```python
from build123d import *

# Parameters (mm, degrees)
SKETCH1_R           = 125
BOSS_EXTRUDE1_DEPTH = 5
SKETCH1_5_R         = 17.5
CUT_EXTRUDE4_DEPTH  = 10


with BuildPart() as part:
    # Sketch1 → Boss-Extrude1 (new body)
    with BuildSketch(Plane(origin=(0, 0, 0), x_dir=(1, 0, 0), z_dir=(0, 1, 0))):
        Circle(SKETCH1_R)
    extrude(amount=BOSS_EXTRUDE1_DEPTH)

    # Sketch1<5> → Cut-Extrude4 (cut)
    with BuildSketch(Plane(origin=(0, 0, 0), x_dir=(1, 0, 0), z_dir=(0, 1, 0))):
        with Locations((25.339393539, 77.986634336)):
            Circle(SKETCH1_5_R)
        with Locations((66.339393539, 48.198390688)):
            Circle(SKETCH1_5_R)
        with Locations((82, 0)):
            Circle(SKETCH1_5_R)
        with Locations((66.339393539, -48.198390688)):
            Circle(SKETCH1_5_R)
        with Locations((25.339393539, -77.986634336)):
            Circle(SKETCH1_5_R)
    extrude(amount=CUT_EXTRUDE4_DEPTH, mode=Mode.SUBTRACT)


solid = part.part
```
Can you work these out from the model? Positions are in its coordinate system, mm. Give positions to 0.01 mm unless a question says otherwise; leave off trailing zeros. Write each loop counter-clockwise with the first axis right and the second up, starting at its lowest first coordinate (ties: lowest second). Pieces come first, ordered by that corner, then holes. Notation, with made-up numbers: (30, -21.75) -> (84, -21.75) arc R18 ccw to (84, -8.75) -> close; hole circle Ø9 at (66, -28). An arc over 180 degrees is marked (long way). One line per item, written item: value.
Q1. Imagine slicing it at B-B on y = 2.95. Please give me the cut outline in (x, z), and give its area (3 significant figures).
Results found:
outline: circle Ø250 at (0, 0); hole circle Ø35 at (25.34, -77.99); hole circle Ø35 at (25.34, 77.99); hole circle Ø35 at (66.34, -48.2); hole circle Ø35 at (66.34, 48.2); hole circle Ø35 at (82, 0)
area: 44,300 mm^2
Q2. For P1, Ø1.5, axis at x = -38, y = 2.5, coming from the -Z side; P2, Ø21, axis at x = 25.34, z = -77.99, coming from the +Y side (3 decimals); P3, Ø3, axis at x = 21, y = 1, coming from the +Z side, each with a flat end and sliding along its axis, tell me the tip position at first contact or that it passes through.
Results found:
P1: stops at z = -119.32
P2: passes through
P3: stops at z = 123.47
Q3. Imagine slicing it at D-D on x = -43. Please give me the cut outline in (y, z).
Results found:
outline: (0, -117.37) -> (5, -117.37) -> (5, 117.37) -> (0, 117.37) -> close
Q4. Please list where these lines run through material, in increasing order: line 1 (X direction, y = 0.6, z = -63); line 2 (Z direction, x = 82, y = 1.2); line 3 (Z direction, x = 55, y = 2.9). Write a range as [from, to].
Results found:
line 1: x = [-107.96, 16.3], [34.38, 57], [75.68, 107.96]
line 2: z = [-94.35, -56.01], [-40.39, -17.5], [17.5, 40.39], [56.01, 94.35]
line 3: z = [-112.25, -61.53], [-34.87, 34.87], [61.53, 112.25]
Q5. We'd pull the mould along X, two halves only. Please class faces 1 (the face through (-124.88, 2.46, -5.5)), 2 (the face through (21.55, 2.46, -60.9)), 3 (the face through (-2, 5, -2)), 4 (the face through (83.03, 2.46, 42.94)): +X half, -X half, draft (parallel to the pull), parting line (faces both ways), or undercut.
Results found:
face 1: parting line
face 2: undercut
face 3: draft
face 4: undercut
Q6. Imagine slicing it at C-C on z = 42. Please give me the cut outline in (x, y).
Results found:
outline: (-117.73, 0) -> (49.97, 0) -> (49.97, 5) -> (-117.73, 5) -> close; (82.7, 0) -> (117.73, 0) -> (117.73, 5) -> (82.7, 5) -> close
Q7. Imagine slicing it at A-A on z = 0. Please give me the cut outline in (x, y), and give its area (4 significant figures).
Results found:
outline: (-125, 0) -> (64.5, 0) -> (64.5, 5) -> (-125, 5) -> close; (99.5, 0) -> (125, 0) -> (125, 5) -> (99.5, 5) -> close
area: 1,075 mm^2
